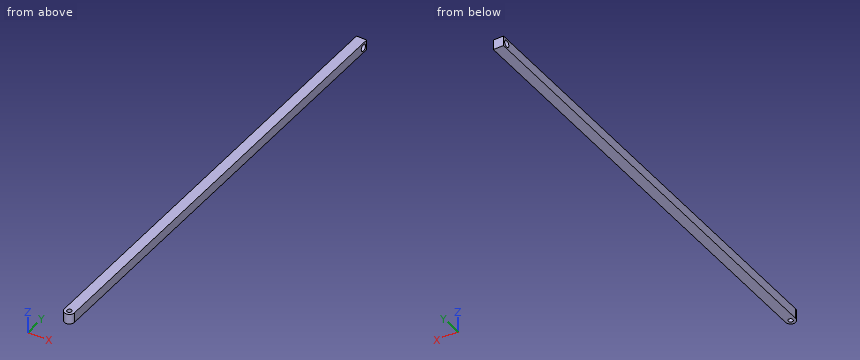
```python
from build123d import *

# Parameters (mm, degrees)
SKETCH1_R           = 0.227761077
BOSS_EXTRUDE1_DEPTH = 1
SKETCH2_R           = 0.323069994
CUT_EXTRUDE1_DEPTH  = 2


with BuildPart() as part:
    # Sketch1 → Boss-Extrude1 (new body)
    with BuildSketch(Plane.XY):
        with BuildLine():
            Line((3.443773372, -22.256132879), (3.443773372, -66.7561317))
            ThreePointArc((3.443773372, -66.7561317), (3.943772783, -67.256132289), (4.443773372, -66.756132879))
            Line((4.443773372, -66.756132879), (4.443773372, -22.256132879))
            Line((4.443773372, -22.256132879), (3.443773372, -22.256132879))
        make_face()
        with Locations((3.943773372, -66.756132289)):
            Circle(SKETCH1_R, mode=Mode.SUBTRACT)
    extrude(amount=BOSS_EXTRUDE1_DEPTH)

    # Sketch2 → Cut-Extrude1 (cut, through all)
    with BuildSketch(Plane(origin=(4.443773372, 0, 0), x_dir=(0, 0, -1), z_dir=(1, 0, 0))):
        with Locations((-0.5, -22.756132879)):
            Circle(SKETCH2_R)
    extrude(amount=-CUT_EXTRUDE1_DEPTH, mode=Mode.SUBTRACT)


solid = part.part
```
The listing builds one solid part. Answer for the finished solid, in the listing's coordinates (mm). Round coordinates to 2 decimals unless told otherwise and drop trailing zeros. Loops run counter-clockwise (first coordinate to the right, second up) from the corner with the lowest first, then second, coordinate; pieces in that order, holes last.
1) A cutting plane is placed at B-B on x = 3.9. Determine the outline of the cut face in (y, z), plus the area to 3 significant figures.
Outcome:
outline: (-67.25, 0) - (-66.98, 0) - (-66.98, 1) - (-67.25, 1) - close; (-66.53, 0) - (-22.26, 0) - (-22.26, 1) - (-66.53, 1) - close; hole circle Ø0.65 at (-22.76, 0.5)
area: 44.2 mm2
2) A cutting plane is placed at A-A on z = 0.5. Determine the outline of the cut face in (x, y), plus the area to 3 significant figures.
Outcome:
outline: (3.44, -66.76) arc R0.5 ccw to (4.44, -66.76) - (4.44, -23.08) - (3.44, -23.08) - close; (3.44, -22.43) - (4.44, -22.43) - (4.44, -22.26) - (3.44, -22.26) - close; hole circle Ø0.46 at (3.94, -66.76)
area: 44.1 mm2
3) Consider line 1 (Y direction, x = 4, z = 0.75); line 2 (Y direction, x = 3.9, z = 0.5); line 3 (Y direction, x = 4.05, z = 0.9). Determine where each line is inside the solid, lowest interval first.
Outcome:
line 1: y = -67.25 to -66.98, -66.54 to -22.96, -22.55 to -22.26
line 2: y = -67.25 to -66.98, -66.53 to -23.08, -22.43 to -22.26
line 3: y = -67.24 to -66.96, -66.55 to -22.26
